from build123d import *

# Parameters (mm, degrees)
SKETCH1_R           = 55
BOSS_EXTRUDE1_DEPTH = 2
SKETCH2_R           = 5
CUT_EXTRUDE1_DEPTH  = 78.807454656
SKETCH4_W           = 25.5
SKETCH4_H           = 56.5
SKETCH4_W_2         = 21.5
SKETCH4_H_2         = 41.5
BOSS_EXTRUDE2_DEPTH = 5
SKETCH5_R           = 1
CUT_EXTRUDE2_DEPTH  = 108.31584226
SKETCH6_W           = 1
SKETCH6_H           = 56.5
CUT_EXTRUDE3_DEPTH  = 1.5


with BuildPart() as part:
    # Sketch1 → Boss-Extrude1 (new body)
    with BuildSketch(Plane(origin=(0, 0, 0), x_dir=(1, 0, 0), z_dir=(0, 1, 0))):
        with Locations(Location((0, 0, 0), (0, 0, 270))):
            Circle(SKETCH1_R)
    extrude(amount=BOSS_EXTRUDE1_DEPTH)

    # Sketch2 → Cut-Extrude1 (cut, through all)
    with BuildSketch(Plane(origin=(0, 2, 0), x_dir=(1, 0, 0), z_dir=(0, 1, 0))):
        with Locations(Location((0, 0, 0), (0, 0, 270))):
            Circle(SKETCH2_R)
    extrude(amount=-CUT_EXTRUDE1_DEPTH, mode=Mode.SUBTRACT)

    # Sketch4 → Boss-Extrude2 (add)
    with BuildSketch(Plane(origin=(16.2, 0, 0), x_dir=(0, 0, -1), z_dir=(1, 0, 0))):
        with Locations((0, 30.25)):
            Rectangle(SKETCH4_W, SKETCH4_H)
        with Locations((0, 30.25)):
            Rectangle(SKETCH4_W_2, SKETCH4_H_2, mode=Mode.SUBTRACT)
    extrude(amount=-BOSS_EXTRUDE2_DEPTH)

    # Sketch5 → Cut-Extrude2 (cut, through all)
    with BuildSketch(Plane(origin=(16.2, 0, 0), x_dir=(0, 0, -1), z_dir=(1, 0, 0))):
        with Locations((-5, 54.3)):
            Circle(SKETCH5_R)
        with Locations((-5, 6.3)):
            Circle(SKETCH5_R)
        with Locations(Location((5, 6.3, 0), (0, 0, 180))):
            Circle(SKETCH5_R)
        with Locations(Location((5, 54.3, 0), (0, 0, 180))):
            Circle(SKETCH5_R)
    extrude(amount=-CUT_EXTRUDE2_DEPTH, mode=Mode.SUBTRACT)

    # Sketch6 → Cut-Extrude3 (cut)
    with BuildSketch(Plane(origin=(16.2, 0, 0), x_dir=(0, 0, -1), z_dir=(1, 0, 0))):
        with Locations((0, 30.25)):
            Rectangle(SKETCH6_W, SKETCH6_H)
    extrude(amount=-CUT_EXTRUDE3_DEPTH, mode=Mode.SUBTRACT)


solid = part.part
Source: CAD feature listing. Evaluate the final solid. Frame: model axes, mm. A direction names the side the tool comes from. Give positions to 0.01 mm unless a question says otherwise; leave off trailing zeros. Write each loop counter-clockwise with the first axis right and the second up, starting at its lowest first coordinate (ties: lowest second). Pieces come first, ordered by that corner, then holes. Notation, with made-up numbers: M 64,32.5 L 100,32.5 A29 ccw 100,65.5 Z; hole C 63,54.25 d1. An arc over 180 degrees is marked long. Return JSON: item names as keys, results as strings. Group by question number.
1) Ray query, L1, parallel to Y at x = 13, z = -5; L2, parallel to X at y = 0.7, z = 0; L3, parallel to Y at x = -43.5, z = -32. Return the intervals inside material, ascending.
2) Cut plane B-B, the plane x = 47.5. Output: boundary loops of the cut face in (y, z).
3) Set-up query: faces 4 (the face through (16.2, 28, -11)), 5 (the face through (11.2, 31, 12)), 6 (the face through (14, 30, -12.75)). Return all of +Z, -Z, +X, -X, +Y, -Y with unobstructed straight access to the full face (end or side cutting, diameter ignored); none if empty.
4) Cut plane C-C, the plane z = 45. Output: boundary loops of the cut face in (x, y).
5) First-contact query: pin 1 Ø2 at (x, z) = (-12, -35.5) entering from +Y; pin 2 Ø2.5 at (y, z) = (6.3, 5) entering from -X; pin 3 Ø1.5 at (x, y) = (14, 30.5) entering from +Z. Flat tips, straight axial feed; report the tip coordinate or a pass-through.
6) Draft query along Z for faces 1 (the face through (14, 30, 10.75)), 2 (the face through (-48.794, 0.986, 25.379)), 3 (the face through (14, 58.5, 0)). Return one class per face: released by +Z, released by -Z, zero draft, split by the parting line, or undercut.
7) Cut plane A-A, the plane y = 17.5. Output: boundary loops of the cut face in (x, z).
Data:
{
 "1": {"L1": "y = 0 to 5.3, 7.3 to 9.5, 51 to 53.3, 55.3 to 58.5", "L2": "x = -55 to -5, 5 to 55", "L3": "y = 0 to 2"},
 "2": {"outline": "M 0,-27.73 L 2,-27.73 L 2,27.73 L 0,27.73 Z"},
 "3": {"face 4": "+Z, -Z, +X, +Y", "face 5": "+Z, -Z, -X, +Y", "face 6": "-Z, +X, -X, +Y"},
 "4": {"outline": "M -31.62,0 L 31.62,0 L 31.62,2 L -31.62,2 Z"},
 "5": {"pin 1": "stops at y = 2", "pin 2": "stops at x = 11.2", "pin 3": "stops at z = 12.75"},
 "6": {"face 1": "undercut", "face 2": "split by the parting line", "face 3": "zero draft"},
 "7": {"outline": "M 11.2,-12.75 L 16.2,-12.75 L 16.2,-10.75 L 11.2,-10.75 Z; M 11.2,10.75 L 16.2,10.75 L 16.2,12.75 L 11.2,12.75 Z"}
}
